Could you check a few things on this model? Use its own coordinates, in mm. Face numbers are marked on the shaded views. Give positions to 0.01 mm unless a question says otherwise; leave off trailing zeros. Loops run counter-clockwise (first coordinate to the right, second up) from the corner with the lowest first, then second, coordinate; pieces in that order, holes last. Notation, with made-up numbers: M 1.5,2.25 L 43.5,2.25 A22 cw 43.5,35.25 Z; hole C 77.5,-0.5 d3. An arc over 180 degrees is marked long. Use CSV: the item, a comma, the result in double quotes.
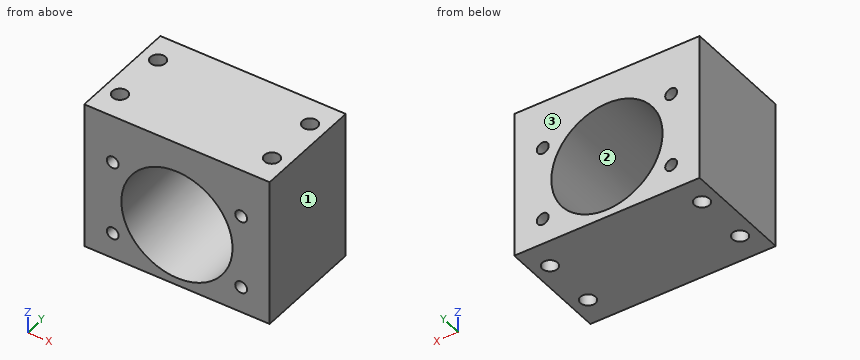
```python
from build123d import *

# Parameters (mm, degrees)
F0_W     = 50
F0_H     = 40
F1_DEPTH = 30
F2_R     = 15
F3_DEPTH = 30.001
F4_D     = 3.2
F6_D     = 4.1


# Not quite as in the source:
# - a feature names something its author has since deleted; it is built from what else it names


with BuildPart() as f1:
    # F0 (on Front) → F1 (new body)
    with BuildSketch(Plane.XZ):
        with Locations((3.412880823, -1.3936108311)):
            Rectangle(F0_W, F0_H)
    extrude(amount=F1_DEPTH)

    # F2 (on face) → F3 (cut, through all)
    with BuildSketch(Plane.XZ.offset(30)):
        with Locations((3.412880823, -4.3936108311)):
            Circle(F2_R)
    extrude(amount=-F3_DEPTH, mode=Mode.SUBTRACT)

    # F4 (through all)
    with Locations(Plane.XZ.offset(30)):
        with Locations((-13.9076272527, -14.3936108311), (-13.9076272527, 5.6063891689), (20.7333888987, 5.6063891689), (20.7333888987, -14.3936108311)):
            Hole(F4_D / 2)

    # F6 (through all)
    with Locations(Plane.XY.offset(18.6063891689)):
        with Locations((23.912880823, -22.5), (23.912880823, -7.5), (-17.087119177, -7.5), (-17.087119177, -22.5)):
            Hole(F6_D / 2)


solid = f1.part
```
1. I want a section at B-B, the plane y = -7.5. List the corners of the cut face in (x, z) for me, then the cut area to 3 significant figures.
Outcome:
outline,"M -21.59,-21.39 L -19.14,-21.39 L -19.14,18.61 L -21.59,18.61 Z; M -15.04,-21.39 L 21.86,-21.39 L 21.86,-15.53 A1.6 cw long 21.86,-13.26 L 21.86,4.47 A1.6 cw long 21.86,6.74 L 21.86,18.61 L -15.04,18.61 L -15.04,6.74 A1.6 cw long -15.04,4.47 L -15.04,-13.26 A1.6 cw long -15.04,-15.53 Z; M 25.96,-21.39 L 28.41,-21.39 L 28.41,18.61 L 25.96,18.61 Z; hole C 3.41,-4.39 d30"
area,"936 mm2"
2. Please list where these lines run through material, in increasing order: line 1 (X direction, y = -24, z = -7.5); line 2 (Z direction, x = 21, y = -7); line 3 (X direction, y = -19, z = -14.5).
Outcome:
line 1,"-21.59 to -18.48, -15.69 to -11.26, 18.09 to 22.52, 25.31 to 28.41"
line 2,"-21.39 to -15.97, -12.82 to 4.03, 7.18 to 18.61"
line 3,"-21.59 to -15.5, -12.31 to -7.67, 14.5 to 19.14, 22.33 to 28.41"
3. If we mould it in two halves opening along X, with no side actions, what happens to the marked faces 1, 2 and 3? For each: +X half, -X half, draft (parallel to the pull), parting line (faces both ways), or undercut.
Outcome:
face 1,"+X half"
face 2,"undercut"
face 3,"draft"
4. I want a section at D-D, the plane x = 20. List the corners of the cut face in (y, z) for me.
Outcome:
outline,"M -30,-21.39 L 0,-21.39 L 0,-15.82 L -30,-15.82 Z; M -30,-12.97 L 0,-12.97 L 0,4.18 L -30,4.18 Z; M -30,7.03 L 0,7.03 L 0,18.61 L -30,18.61 Z"
5. I want a section at C-C, the plane x = 9.5. List the corners of the cut face in (y, z) for me.
Outcome:
outline,"M -30,-21.39 L 0,-21.39 L 0,-18.1 L -30,-18.1 Z; M -30,9.32 L 0,9.32 L 0,18.61 L -30,18.61 Z"
6. I'm going to push a flat-ended pin straight in: pin 1 Ø2 at (x, z) = (-0.5, 8.5) entering from +Y. Where does the tip first touch, or does it pass through?
Outcome:
pin 1,"through"
7. I want a section at A-A, the plane z = -7.5. List the corners of the cut face in (x, y) for me, then the cut area to 3 significant figures.
Outcome:
outline,"M -21.59,-30 L -11.26,-30 L -11.26,0 L -21.59,0 Z; M 18.09,-30 L 28.41,-30 L 28.41,0 L 18.09,0 Z; hole C -17.09,-22.5 d4.1; hole C -17.09,-7.5 d4.1; hole C 23.91,-22.5 d4.1; hole C 23.91,-7.5 d4.1"
area,"567 mm2"
